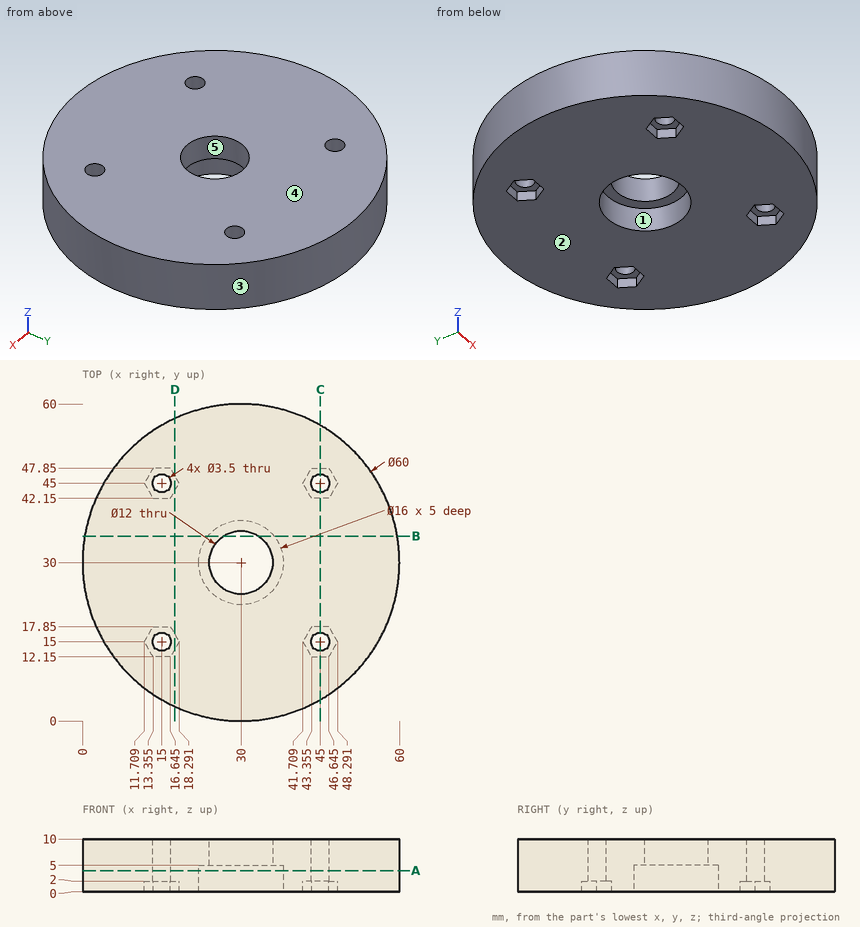
The figure shows three views and two pictorial views of one solid part (mm, origin at its lowest corner). Answer the questions. A direction names the side the tool comes from. Coordinates: 2 decimals unless noted, no trailing zeros. Loops run counter-clockwise (first coordinate to the right, second up) from the corner with the lowest first, then second, coordinate; pieces in that order, holes last.
1) Find the intervals of material crossed by L1, parallel to Y at x = 30, z = 2.85; L2, parallel to Y at x = 30, z = 7.9; L3, parallel to X at y = 34.5, z = 2.5 (1 decimal), in increasing order.
2) Find section C-C on x = 45. Write down the section's boundary in (y, z), then the cut area to 3 significant figures.
3) Flat-ended cylindrical pins translate along their axes: pin 1 Ø3 at (x, y) = (45.5, 16) entering from -Z; pin 2 Ø5 at (y, z) = (53.5, 1.5) entering from +X (1 decimal); pin 3 Ø4 at (x, z) = (43.5, 8) entering from +Y; pin 4 Ø9.5 at (x, y) = (30, 30) entering from +Z. Find the tip coordinate at first contact, or state that the pin passes through.
4) Determine the mould class of the marked faces 3, 4 and 5 for opening direction Y: pulls with the +Y half, pulls with the -Y half, needs draft (parallel to the pull), parting line crosses it, or undercut.
5) Find section D-D on x = 17.5. Write down the section's boundary in (y, z).
6) Find section B-B on y = 35. Write down the section's boundary in (x, z) (1 decimal).
7) Find section A-A on z = 4. Write down the section's boundary in (x, y).
8) A tool of negligible diameter and unlimited length cuts with its end or side. For the marked faces 1 and 2, from which of +Z, -Z, +X, -X, +Y, -Y can it reach the whole face along a straight path? Write none if from no direction.
Values:
1. L1: y = 0 to 22, 38 to 60
1. L2: y = 0 to 24, 36 to 60
1. L3: x = 0.3 to 23.4, 36.6 to 59.7
2. outline: (4.02, 0) - (12.15, 0) - (12.15, 2) - (13.25, 2) - (13.25, 10) - (4.02, 10) - close; (16.75, 2) - (17.85, 2) - (17.85, 0) - (42.15, 0) - (42.15, 2) - (43.25, 2) - (43.25, 10) - (16.75, 10) - close; (46.75, 2) - (47.85, 2) - (47.85, 0) - (55.98, 0) - (55.98, 10) - (46.75, 10) - close
2. area: 441 mm2
3. pin 1: stops at z = 2
3. pin 2: stops at x = 51.4
3. pin 3: stops at y = 57.71
3. pin 4: passes through
4. face 3: parting line crosses it
4. face 4: needs draft
4. face 5: undercut
5. outline: (2.73, 0) - (13.63, 0) - (13.63, 2) - (16.37, 2) - (16.37, 0) - (43.63, 0) - (43.63, 2) - (46.37, 2) - (46.37, 0) - (57.27, 0) - (57.27, 10) - (2.73, 10) - close
6. outline: (0.4, 0) - (23.8, 0) - (23.8, 5) - (26.7, 5) - (26.7, 10) - (0.4, 10) - close; (33.3, 5) - (36.2, 5) - (36.2, 0) - (59.6, 0) - (59.6, 10) - (33.3, 10) - close
7. outline: circle Ø60 at (30, 30); hole circle Ø3.5 at (15, 15); hole circle Ø3.5 at (15, 45); hole circle Ø16 at (30, 30); hole circle Ø3.5 at (45, 15); hole circle Ø3.5 at (45, 45)
8. face 1: -Z
8. face 2: -Z, +X, -X, +Y, -Y
